Design review of the part built by this model. Coordinates are the model's own, in mm. A direction names the side the tool comes from. Round coordinates to 2 decimals unless told otherwise and drop trailing zeros. Order: outer loops, then holes, each group sorted by start corner. A loop starts at its lowest first (then second) coordinate and runs counter-clockwise, first axis right, second up. Notation, with made-up numbers: M 20.25,-26.5 L 71.25,-26.5 A27 cw 71.25,8.5 Z; hole C 19.5,45.5 d9. An arc over 180 degrees is marked long. Use a Markdown table: item, result. Add a question column.
(1) To check wall thickness, follow probe 1 along Y at (x, z) = (58.5, -4); probe 2 along Z at (x, y) = (53, 15.5); probe 3 along Y at (x, z) = (41, -43). State the ranges of each line that lie inside material, in increasing order. Write a range as from..to.
(2) Take a section at B-B (y = 9.75). Write out the cut boundary in (x, z).
(3) Take a section at C-C (x = 31). Write out the cut boundary in (y, z), then the cut area to 3 significant figures.
(4) The part is to be moulded in two halves that separate along X. For faces 1 (the face through (20.8, 4, -25)), 2 (the face through (5.9, 5.14, -24.65)), 3 (the face through (22.27, 4.48, -19.25)), 4 (the face through (56.06, 15.04, -43.69)), say which applies: released by +X, released by -X, zero draft, split by the parting line, or undercut.
(5) Machinability: for faces 5 (the face through (60, 4, -31)), 6 (the face through (35.73, 4.48, -30.75)), 7 (the face through (42, 3, -25)), which of the approach directions +Z, -Z, +X, -X, +Y, -Y give a long, thin tool a straight path to every point of the face, cutting with its end or side? Answer none if there is none.
(6) For pin 1 (4 mm diameter, centred on y = 12, z = -5, fed in from -X); pin 2 (3 mm diameter, centred on x = 31, z = -16, fed in from -Y); pin 3 (2.5 mm diameter, centred on y = 1, z = -26, fed in from +X), all flat-tipped, find the tip position at first contact; note any pin that passes through.
(7) Take a section at A-A (z = -46). Write out the cut boundary in (x, y).
(8) Take a section at D-D (y = 16). Write out the cut boundary in (x, z), then the cut area to 3 significant figures.
```python
from build123d import *

# Parameters (mm, degrees)
SKETCH1_W           = 60
SKETCH1_H           = 50
BOSS_EXTRUDE1_DEPTH = 6
SKETCH2_W           = 8
SKETCH2_H           = 8
BOSS_EXTRUDE2_DEPTH = 20
CUT_EXTRUDE1_REACH  = 84.316
SKETCH3_R           = 2.5
SKETCH4_W           = 28
SKETCH4_H           = 28
SKETCH4_W_2         = 17
CUT_EXTRUDE2_DEPTH  = 3
CUT_EXTRUDE3_REACH  = 83.419
SKETCH5_R           = 1.85
SKETCH6_W           = 50
SKETCH6_H           = 6
CUT_EXTRUDE4_DEPTH  = 5
FILLET1_R           = 1
FILLET2_R           = 1
FILLET4_R           = 3


with BuildPart() as part:
    # Sketch1 → Boss-Extrude1 (new body)
    with BuildSketch(Plane(origin=(0, 0, 0), x_dir=(1, 0, 0), z_dir=(0, 1, 0))):
        with Locations((30, 25)):
            Rectangle(SKETCH1_W, SKETCH1_H)
    extrude(amount=BOSS_EXTRUDE1_DEPTH)

    # Sketch2 → Boss-Extrude2 (add)
    with BuildSketch(Plane(origin=(0, 6, 0), x_dir=(1, 0, 0), z_dir=(0, 1, 0))):
        with Locations((56, 4)):
            Rectangle(SKETCH2_W, SKETCH2_H)
    boss_extrude2 = extrude(amount=BOSS_EXTRUDE2_DEPTH)

    # Sketch3 → Cut-Extrude1 (cut, up to next)
    with BuildSketch(Plane(origin=(60, 0, 0), x_dir=(0, 0, -1), z_dir=(1, 0, 0)), mode=Mode.PRIVATE) as cut_extrude1_sk1:
        with Locations((4, 16)):
            Circle(SKETCH3_R)
    cut_extrude1_tool1 = extrude(cut_extrude1_sk1.sketch, amount=-CUT_EXTRUDE1_REACH, mode=Mode.PRIVATE) & part.part
    cut_extrude1 = cut_extrude1_tool1.solids().sort_by_distance((60, 16, -4))[0]
    add(cut_extrude1, mode=Mode.SUBTRACT)

    # Mirror1: Boss-Extrude2, Cut-Extrude1 across plane
    add(boss_extrude2.mirror(Plane.XY.offset(-25)))
    add(cut_extrude1.mirror(Plane.XY.offset(-25)), mode=Mode.SUBTRACT)

    # Sketch4 → Cut-Extrude2 (cut)
    with BuildSketch(Plane.XZ):
        with Locations((29, -25)):
            Rectangle(SKETCH4_W, SKETCH4_H)
        with Locations((51.5, -25)):
            Rectangle(SKETCH4_W_2, SKETCH4_H)
    extrude(amount=-CUT_EXTRUDE2_DEPTH, mode=Mode.SUBTRACT)

    # Sketch5 → Cut-Extrude3 (cut, up to next)
    with BuildSketch(Plane.XZ.offset(-3), mode=Mode.PRIVATE) as cut_extrude3_sk1:
        with Locations(Location((20.5, -16.5, 0), (0, 0, 270))):
            Circle(SKETCH5_R)
    cut_extrude3_tool1 = extrude(cut_extrude3_sk1.sketch, amount=-CUT_EXTRUDE3_REACH, mode=Mode.PRIVATE) & part.part
    # Sketch5 → Cut-Extrude3 (cut, up to next)
    with BuildSketch(Plane.XZ.offset(-3), mode=Mode.PRIVATE) as cut_extrude3_sk2:
        with Locations(Location((37.5, -16.5, 0), (0, 0, 270))):
            Circle(SKETCH5_R)
    cut_extrude3_tool2 = extrude(cut_extrude3_sk2.sketch, amount=-CUT_EXTRUDE3_REACH, mode=Mode.PRIVATE) & part.part
    # Sketch5 → Cut-Extrude3 (cut, up to next)
    with BuildSketch(Plane.XZ.offset(-3), mode=Mode.PRIVATE) as cut_extrude3_sk3:
        with Locations(Location((37.5, -33.5, 0), (0, 0, 270))):
            Circle(SKETCH5_R)
    cut_extrude3_tool3 = extrude(cut_extrude3_sk3.sketch, amount=-CUT_EXTRUDE3_REACH, mode=Mode.PRIVATE) & part.part
    # Sketch5 → Cut-Extrude3 (cut, up to next)
    with BuildSketch(Plane.XZ.offset(-3), mode=Mode.PRIVATE) as cut_extrude3_sk4:
        with Locations(Location((20.5, -33.5, 0), (0, 0, 270))):
            Circle(SKETCH5_R)
    cut_extrude3_tool4 = extrude(cut_extrude3_sk4.sketch, amount=-CUT_EXTRUDE3_REACH, mode=Mode.PRIVATE) & part.part
    # Sketch5 → Cut-Extrude3 (cut, up to next)
    with BuildSketch(Plane.XZ.offset(-3), mode=Mode.PRIVATE) as cut_extrude3_sk5:
        with BuildLine():
            Line((37.2, -20.75), (37.2, -29.25))
            ThreePointArc((37.2, -29.25), (35.7, -30.75), (34.2, -29.25))
            Line((34.2, -29.25), (34.2, -20.75))
            ThreePointArc((34.2, -20.75), (35.7, -19.25), (37.2, -20.75))
        make_face()
    cut_extrude3_tool5 = extrude(cut_extrude3_sk5.sketch, amount=-CUT_EXTRUDE3_REACH, mode=Mode.PRIVATE) & part.part
    # Sketch5 → Cut-Extrude3 (cut, up to next)
    with BuildSketch(Plane.XZ.offset(-3), mode=Mode.PRIVATE) as cut_extrude3_sk6:
        with BuildLine():
            Line((23.8, -20.75), (23.8, -29.25))
            ThreePointArc((23.8, -29.25), (22.3, -30.75), (20.8, -29.25))
            Line((20.8, -29.25), (20.8, -20.75))
            ThreePointArc((20.8, -20.75), (22.3, -19.25), (23.8, -20.75))
        make_face()
    cut_extrude3_tool6 = extrude(cut_extrude3_sk6.sketch, amount=-CUT_EXTRUDE3_REACH, mode=Mode.PRIVATE) & part.part
    add(cut_extrude3_tool1.solids().sort_by_distance((20.5, 3, -16.5))[0], mode=Mode.SUBTRACT)
    add(cut_extrude3_tool2.solids().sort_by_distance((37.5, 3, -16.5))[0], mode=Mode.SUBTRACT)
    add(cut_extrude3_tool3.solids().sort_by_distance((37.5, 3, -33.5))[0], mode=Mode.SUBTRACT)
    add(cut_extrude3_tool4.solids().sort_by_distance((20.5, 3, -33.5))[0], mode=Mode.SUBTRACT)
    add(cut_extrude3_tool5.solids().sort_by_distance((35.7, 3, -25))[0], mode=Mode.SUBTRACT)
    add(cut_extrude3_tool6.solids().sort_by_distance((22.3, 3, -25))[0], mode=Mode.SUBTRACT)

    # Sketch6 → Cut-Extrude4 (cut)
    with BuildSketch(Plane.ZY):
        with Locations((-25, 3)):
            Rectangle(SKETCH6_W, SKETCH6_H)
    extrude(amount=-CUT_EXTRUDE4_DEPTH, mode=Mode.SUBTRACT)

    # Fillet1
    fillet1_edges = [part.edges().sort_by_distance(p)[0] for p in [
        (56, 26, -8),
        (56, 26, 0),
        (56, 26, -50),
        (56, 26, -42),
    ]]
    fillet(fillet1_edges, radius=FILLET1_R)

    # Fillet2
    fillet2_edges = [part.edges().sort_by_distance(p)[0] for p in [
        (56, 6, -8),
        (52, 6, -4),
        (56, 6, -42),
        (52, 6, -46),
    ]]
    fillet(fillet2_edges, radius=FILLET2_R)

    # Fillet4
    fillet4_edges = [part.edges().sort_by_distance(p)[0] for p in [
        (5, 6, -25),
    ]]
    fillet(fillet4_edges, radius=FILLET4_R)


solid = part.part
```
Verdict:
| question | item | result |
|---|---|---|
| 1 | probe 1 | y = 0..13.5, 18.5..26 |
| 1 | probe 2 | z = -50..-48.45, -43.55..-42, -8..-6.45, -1.55..0 |
| 1 | probe 3 | y = 0..6 |
| 2 | outline | M 52,-50 L 60,-50 L 60,-42 L 52,-42 Z; M 52,-8 L 60,-8 L 60,0 L 52,0 Z |
| 3 | outline | M 0,-50 L 6,-50 L 6,0 L 0,0 L 0,-11 L 3,-11 L 3,-39 L 0,-39 Z |
| 3 | area | 216 mm^2 |
| 4 | face 1 | undercut |
| 4 | face 2 | released by -X |
| 4 | face 3 | undercut |
| 4 | face 4 | zero draft |
| 5 | face 5 | +Z, -Z, +X, +Y, -Y |
| 5 | face 6 | +Y, -Y |
| 5 | face 7 | +X, -Y |
| 6 | pin 1 | stops at x = 52 |
| 6 | pin 2 | stops at y = 3 |
| 6 | pin 3 | stops at x = 15 |
| 7 | outline | M 5,0 L 60,0 L 60,13.5 L 52,13.5 L 52,7 A1 cw 51,6 L 8,6 A3 ccw 5,3 Z; M 52,18.5 L 60,18.5 L 60,26 L 52,26 Z |
| 8 | outline | M 52,-50 L 60,-50 L 60,-48.5 L 52,-48.5 Z; M 52,-43.5 L 60,-43.5 L 60,-42 L 52,-42 Z; M 52,-8 L 60,-8 L 60,-6.5 L 52,-6.5 Z; M 52,-1.5 L 60,-1.5 L 60,0 L 52,0 Z |
| 8 | area | 48.0 mm^2 |
